Geometry check sheet. Reference: the model listing, model coordinates, mm. A direction names the side the tool comes from. Coordinates: 2 decimals unless noted, no trailing zeros. Write each loop counter-clockwise with the first axis right and the second up, starting at its lowest first coordinate (ties: lowest second). Pieces come first, ordered by that corner, then holes.
from build123d import *

# Parameters (mm, degrees)
SKETCH1_R           = 5.2
SKETCH1_R_2         = 4.2
BOSS_EXTRUDE2_DEPTH = 27
SKETCH1_3_R         = 6.2
SKETCH1_3_R_2       = 5.2
BOSS_EXTRUDE3_DEPTH = 21
CUT_EXTRUDE1_START  = 27
SKETCH3_W           = 6.6
SKETCH3_H           = 6.6
CUT_EXTRUDE1_DEPTH  = 15
CUT_EXTRUDE2_START  = -27
SKETCH3_3_W         = 6.6
SKETCH3_3_H         = 6.6
CUT_EXTRUDE2_DEPTH  = 15


with BuildPart() as part:
    # Sketch1 → Boss-Extrude2 (new, symmetric)
    with BuildSketch(Plane.XY):
        Circle(SKETCH1_R)
        Circle(SKETCH1_R_2, mode=Mode.SUBTRACT)
    extrude(amount=BOSS_EXTRUDE2_DEPTH, both=True)

    # Sketch1<3> → Boss-Extrude3 (add, symmetric)
    with BuildSketch(Plane.XY):
        with Locations(Location((0, 0, 0), (0, 0, 180))):
            Circle(SKETCH1_3_R)
        Circle(SKETCH1_3_R_2, mode=Mode.SUBTRACT)
    extrude(amount=BOSS_EXTRUDE3_DEPTH, both=True)

    # Sketch3 → Cut-Extrude1 (cut)
    with BuildSketch(Plane.XY.offset(CUT_EXTRUDE1_START)):
        Rectangle(SKETCH3_W, SKETCH3_H)
    extrude(amount=-CUT_EXTRUDE1_DEPTH, mode=Mode.SUBTRACT)

    # Sketch3<3> → Cut-Extrude2 (cut)
    with BuildSketch(Plane.XY.offset(CUT_EXTRUDE2_START)):
        Rectangle(SKETCH3_3_W, SKETCH3_3_H)
    extrude(amount=CUT_EXTRUDE2_DEPTH, mode=Mode.SUBTRACT)


solid = part.part
1. Draft check along X on faces 3 (the flat face through (0.7, 4.3, 27)), 4 (the cylindrical face through (-0.677, 5.156, -23.958)), 5 (the cylindrical face through (3.88, -1.61, -0.38)). Enter one of: released by +X, released by -X, zero draft, split by the parting line, or undercut.
Computed values:
face 3: zero draft
face 4: split by the parting line
face 5: undercut
2. Access from +Z, -Z, +X, -X, +Y, -Y to the whole of each face (thin tool, end or side, straight path). Record for faces 1 (the cylindrical face through (-0.677, 5.156, 24.042)), 2 (the cylindrical face through (-5.9, -1.9, 0.3)).
Computed values:
face 1: +Z
face 2: +Z, -Z
3. Sectioned sample at D-D, the plane z = 0. Record the boundary of the cut face in (x, y).
Computed values:
outline: circle Ø12.4 at (0, 0); hole circle Ø8.4 at (0, 0)
4. Sectioned sample at A-A, the plane x = 0. Record the boundary of the cut face in (y, z).
Computed values:
outline: (-6.2, -21) - (-5.2, -21) - (-5.2, -27) - (-4.2, -27) - (-4.2, 27) - (-5.2, 27) - (-5.2, 21) - (-6.2, 21) - close; (4.2, -27) - (5.2, -27) - (5.2, -21) - (6.2, -21) - (6.2, 21) - (5.2, 21) - (5.2, 27) - (4.2, 27) - close
5. Sectioned sample at C-C, the plane z = 24.5. Record the boundary of the cut face in (x, y), and give its area (3 significant figures).
Computed values:
outline: circle Ø10.4 at (0, 0); hole (-3.3, -3.3) - (-2.6, -3.3) arc R4.2 ccw to (2.6, -3.3) - (3.3, -3.3) - (3.3, -2.6) arc R4.2 ccw to (3.3, 2.6) - (3.3, 3.3) - (2.6, 3.3) arc R4.2 ccw to (-2.6, 3.3) - (-3.3, 3.3) - (-3.3, 2.6) arc R4.2 ccw to (-3.3, -2.6) - close
area: 28.6 mm2
6. Gauge pin test, flat ends, axial feed: pin 1 Ø5 at (y, z) = (3.5, 7.5) entering from -X; pin 2 Ø0.8 at (x, z) = (-3, 19) entering from -Y; pin 3 Ø0.8 at (x, z) = (3, -23) entering from -Y. Record the tip position at first contact, or that the pin passes through.
Computed values:
pin 1: stops at x = -6.12
pin 2: stops at y = -5.63
pin 3: stops at y = -4.5
7. Thickness scan on line 1 along Y through (x, z) = (0, -7); line 2 along X through (y, z) = (2.75, -10); line 3 along Y through (x, z) = (2, 10). Record the ranges inside material, lowest first.
Computed values:
line 1: y = -6.2 to -4.2, 4.2 to 6.2
line 2: x = -5.56 to -3.17, 3.17 to 5.56
line 3: y = -5.87 to -3.69, 3.69 to 5.87
